The model under review builds one solid part; all positions refer to its coordinate system, in mm. Give positions to 0.01 mm unless a question says otherwise; leave off trailing zeros. Loops run counter-clockwise (first coordinate to the right, second up) from the corner with the lowest first, then second, coordinate; pieces in that order, holes last. Notation, with made-up numbers: (-33, -31.5) - (7, -31.5) arc R26 cw to (7, -12.5) - close; hole circle Ø11 at (5.5, -20.5). An arc over 180 degrees is marked (long way). Answer as a JSON object with one key per item and string values.
Autodesk Inventor part; units mm, degrees
ref_plane "YZ Plane" through (0, 0, 0) normal (1, 0, 0) x (0, 1, 0)
ref_plane "XZ Plane" through (0, 0, 0) normal (0, 1, 0) x (-1, 0, 0)
ref_plane "XY Plane" through (0, 0, 0) normal (0, 0, 1) x (1, 0, 0)
sketch "Sketch1" plane through (0, 0, 0) normal (0, 1, 0) x (-1, 0, 0)
  line L0 (0, 0) -> (66.04, 0)
  line L1 (66.04, 0) -> (66.04, -81.915)
  line L2 (66.04, -81.915) -> (0, -81.915)
  line L3 (0, -81.915) -> (0, 0)
  dimension "d0" = 66.04
  dimension "d1" = 81.915
extrude "Extrusion1" add sketch "Sketch1" along normal blind 6.35
fillet "Fillet1" radius 3.175 4 edges at (0, 3.175, 0) (-66.04, 3.175, 0) (0, 3.175, -81.915) (-66.04, 3.175, -81.915)
fillet "Fillet2" radius 3.175 8 edges at (-0.9299, 6.35, -80.9851) (-33.02, 6.35, -81.915) (-65.1101, 6.35, -80.9851) (-66.04, 6.35, -40.9575) (-65.1101, 6.35, -0.9299) (-33.02, 6.35, 0) (-0.9299, 6.35, -0.9299) (0, 6.35, -40.9575)
sketch "Sketch2" plane through (0, 6.35, 0) normal (0, 1, 0) x (1, 0, 0)
  line L0 (0, 0) -> (0, 23.0418) construction
  line L1 (0, 78.74) -> (0, 3.175)
  line L2 (0, 0) -> (-15.3745, 0) construction
  line L3 (-3.175, 0) -> (-62.865, 0)
  line L4 (0, 2.3813) -> (-36.1213, 2.3813) construction
  line L5 (-33.02, 0) -> (-33.02, 49.3607) construction
  circle A0 centre (-7.62, 2.3813) radius 1.632
  line L6 (-3.175, 78.74) -> (-3.175, 3.175)
  line L7 (-3.175, 40.9575) -> (-28.1102, 40.9575) construction
  circle A1 centre (-58.42, 2.3813) radius 1.632
  circle A2 centre (-7.62, 79.5337) radius 1.632
  circle A3 centre (-58.42, 79.5337) radius 1.632
  dimension "d6" = 2.3813
  dimension "d7" = 3.2639
  dimension "d8" = 25.4
extrude "Extrusion2" cut sketch "Sketch2" against normal blind 6.35
properties part number "top"
Q1. Clearance check with flat-ended pins moving along their axes: pin 1 Ø1 at (x, y) = (-24, 5) entering from -Z; pin 2 Ø2 at (x, z) = (-7.62, -79.53) entering from -Y. State where each tip first meets the part, or that it passes through.
Results:
{"pin 1": "stops at z = -81.63", "pin 2": "passes through"}
Q2. The part is to be moulded in two halves that separate along Z. For faces 1 (the face through (-6.867, 3.219, -78.086)), 2 (the face through (-32.602, 5.395, -81.01)), 3 (the face through (-33, 2, 0)), say which applies: +Z half, -Z half, draft (parallel to the pull), parting line (faces both ways), or undercut.
Results:
{"face 1": "undercut", "face 2": "-Z half", "face 3": "+Z half"}
Q3. Consider section A-A, the plane x = -7.62. State the section outline as (y, z) points (3 decimals).
Results:
{"outline": "(0, -81.915) - (3.175, -81.915) arc R3.175 ccw to (5.224, -81.166) - (0, -81.166) - close; (0, -77.902) - (6.35, -77.902) - (6.35, -4.013) - (0, -4.013) - close; (0, -0.749) - (5.224, -0.749) arc R3.175 ccw to (3.175, 0) - (0, 0) - close"}
Q4. To check wall thickness, follow probe 1 along Z at (x, y) = (-7.62, 1.5) (3 decimals); probe 2 along Z at (x, y) = (-7.62, 4.75); probe 3 along Z at (x, y) = (-25, 3.25). State the ranges of each line that lie inside material, in increasing order. Write a range as [from, to].
Results:
{"probe 1": "z = [-81.915, -81.166], [-77.902, -4.013], [-0.749, 0]", "probe 2": "z = [-81.5, -81.17], [-77.9, -4.01], [-0.75, -0.42]", "probe 3": "z = [-81.91, 0]"}
